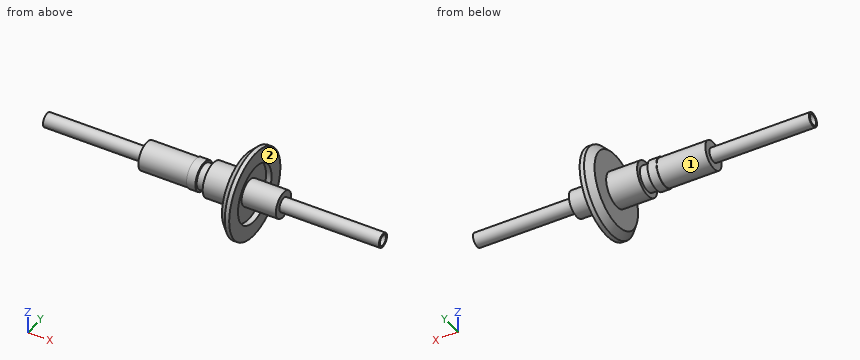
```python
from build123d import *


with BuildPart() as part:
    # Axial profile (mm) → Full revolution (revolve)
    with BuildSketch(Plane.XY, mode=Mode.PRIVATE) as full_revolution_sk:
        Polygon((-94, 2.4), (58, 2.4), (58, 3.2), (13, 3.2), (13, 6), (-2.5, 6), (-2.5, 13.1), (0, 13.1), (0, 20), (-2, 20), (-5, 17), (-5, 7.9), (-19, 7.9), (-19, 5.7), (-23, 5.7), (-23, 6.7), (-27, 6.7), (-27, 6.4), (-49, 6.4), (-49, 3.2), (-94, 3.2), align=None)
    revolve(full_revolution_sk.sketch.rotate(Axis((-110, 0, 0), (1, 0, 0)), 90), axis=Axis((-110, 0, 0), (1, 0, 0)))


solid = part.part
```
Input: part model. Units: mm. Frame: model coordinates. Face numbers are marked on the shaded views. A direction names the side the tool comes from. Coordinates: 2 decimals unless noted, no trailing zeros. Write each loop counter-clockwise with the first axis right and the second up, starting at its lowest first coordinate (ties: lowest second). Pieces come first, ordered by that corner, then holes. Notation, with made-up numbers: (76.25, 81) -> (102.25, 81) arc R15 cw to (102.25, 87) -> close; hole circle Ø7 at (33, 59.25). An arc over 180 degrees is marked (long way). Answer as a JSON object with one key per item and string values.
1. First-contact query: P1, Ø1, axis at x = -73.5, z = 0.5, coming from the -Y side; P2, Ø6, axis at y = 15.5, z = 15, coming from the +X side; P3, Ø8, axis at y = 10.5, z = 6.5, coming from the -X side. Flat tips, straight axial feed; report the tip coordinate or a pass-through.
Result set:
{"P1": "stops at y = -3.2", "P2": "stops at x = 0", "P3": "stops at x = -5"}
2. Section A-A on x = -51.5. Return the cut outline in (y, z), then the cut area to 3 significant figures.
Result set:
{"outline": "circle Ø6.4 at (0, 0); hole circle Ø4.8 at (0, 0)", "area": "14.1 mm2"}
3. Access query for the marked faces 1 and 2. Directions: +Z, -Z, +X, -X, +Y, -Y. A direction counts if a zero-diameter tool reaches every point of the face in a straight line with its end or side. Return the directions, or none.
Result set:
{"face 1": "-X", "face 2": "+X"}
4. Material intervals for line 1 (Y direction, x = -1.7, z = 0); line 2 (Y direction, x = -23.5, z = 0); line 3 (X direction, y = -2, z = -8), sorted ascending. Write a range as from..to.
Result set:
{"line 1": "y = -20..-13.1, -6..-2.4, 2.4..6, 13.1..20", "line 2": "y = -6.7..-2.4, 2.4..6.7", "line 3": "x = -5..-2.5"}
